```python
from build123d import *

# Parameters (mm, degrees)
P_IDAT_VYSUNUT_M1_DEPTH = 8
ZAOBLIT1_R              = 2


with BuildPart() as part:
    # Skica1 → Přidat vysunutím1 (new body)
    with BuildSketch(Plane.XY):
        with BuildLine():
            Line((1.2, 7.9), (1.2, 5.9))
            Line((1.2, 5.9), (3, 5.9))
            Line((3, 5.9), (3, 4.1))
            Line((3, 4.1), (1.2, 4.1))
            Line((1.2, 4.1), (1.2, -4.1))
            Line((1.2, -4.1), (3, -4.1))
            Line((3, -4.1), (3, -5.9))
            Line((3, -5.9), (1.2, -5.9))
            Line((1.2, -5.9), (1.2, -7.9))
            Line((1.2, -7.9), (-0.9, -7.9))
            Line((-0.9, -7.9), (-0.9, -9.7))
            Line((-0.9, -9.7), (-2.7, -9.7))
            Line((-2.7, -9.7), (-2.7, -7.9))
            Line((-2.7, -7.9), (-4.526252218, -7.9))
            ThreePointArc((-4.526252218, -7.9), (-4.233358999, -7.192893219), (-3.526252218, -6.9))
            ThreePointArc((-3.526252218, -6.9), (-2.970681985, -6.731469612), (-2.602372686, -6.282683432))
            Line((-2.602372686, -6.282683432), (0, 0))
            Line((0, 0), (-2.602372686, 6.282683432))
            ThreePointArc((-2.602372686, 6.282683432), (-2.970681985, 6.731469612), (-3.526252218, 6.9))
            ThreePointArc((-3.526252218, 6.9), (-4.233358999, 7.192893219), (-4.526252218, 7.9))
            Line((-4.526252218, 7.9), (-2.7, 7.9))
            Line((-2.7, 7.9), (-2.7, 9.7))
            Line((-2.7, 9.7), (-0.9, 9.7))
            Line((-0.9, 9.7), (-0.9, 7.9))
            Line((-0.9, 7.9), (1.2, 7.9))
        make_face()
    extrude(amount=P_IDAT_VYSUNUT_M1_DEPTH)

    # Zaoblit1
    zaoblit1_edges = [part.edges().sort_by_distance(p)[0] for p in [
        (0, 0, 4),
    ]]
    fillet(zaoblit1_edges, radius=ZAOBLIT1_R)


solid = part.part
```
For this review, take the finished solid that the model builds, in its own axes (mm). A direction names the side the tool comes from. Give positions to 0.01 mm unless a question says otherwise; leave off trailing zeros. Write each loop counter-clockwise with the first axis right and the second up, starting at its lowest first coordinate (ties: lowest second). Pieces come first, ordered by that corner, then holes.
Item 1: Take a section at A-A (x = 2.75). Give the boundary of the cut face in (y, z).
Item 2: Wall thickness on probe 1 along Y at (x, z) = (2.5, 1.5); probe 2 along Y at (x, z) = (0.25, 6.25); probe 3 along X at (y, z) = (-9, 1.5): over which ranges is each line inside the solid? List them lowest first.
Item 3: Take a section at B-B (z = 2.75). Give the boundary of the cut face in (x, y), and give its area (3 significant figures).
Item 4: Machinability: for faces 5 (the face through (1.2, 7, 4)), 6 (the face through (-2.7, -9, 4)), 7 (the face through (1.2, -7, 4)), 8 (the face through (-1.476, -3.563, 3.944)), which of the approach directions +Z, -Z, +X, -X, +Y, -Y give a long, thin tool a straight path to every point of the face, cutting with its end or side? Answer none if there is none.
Item 5: Insertion check: P1, Ø1.4, axis at x = 2, z = 5, coming from the +Y side; P2, Ø4, axis at x = 2, z = 2, coming from the -Y side; P3, Ø2, axis at y = 9, z = 5, coming from the -X side; P4, Ø4, axis at x = -3.5, z = 4.5, coming from the +Y side. Each pin has a flat end and moves straight along its axis. Give the tip position at first contact, or say it passes through.
Item 6: Take a section at D-D (y = -1). Give the boundary of the cut face in (x, z), and give its area (3 significant figures).
Item 7: Take a section at C-C (x = -3.25). Give the boundary of the cut face in (y, z).
Item 8: The part is to be moulded in two halves that separate along Y. For faces 1 (the face through (0, -7.9, 4)), 2 (the face through (1.2, 0, 4)), 3 (the face through (0, 0, 0)), 4 (the face through (-0.165, -0.011, 4.056)), say which applies: +Y half, -Y half, draft (parallel to the pull), parting line (faces both ways), or undercut.
Established:
1. outline: (-5.9, 0) - (-4.1, 0) - (-4.1, 8) - (-5.9, 8) - close; (4.1, 0) - (5.9, 0) - (5.9, 8) - (4.1, 8) - close
2. probe 1: y = -5.9 to -4.1, 4.1 to 5.9
2. probe 2: y = -7.9 to 7.9
2. probe 3: x = -2.7 to -0.9
3. outline: (-4.53, -7.9) - (-2.7, -7.9) - (-2.7, -9.7) - (-0.9, -9.7) - (-0.9, -7.9) - (1.2, -7.9) - (1.2, -5.9) - (3, -5.9) - (3, -4.1) - (1.2, -4.1) - (1.2, 4.1) - (3, 4.1) - (3, 5.9) - (1.2, 5.9) - (1.2, 7.9) - (-0.9, 7.9) - (-0.9, 9.7) - (-2.7, 9.7) - (-2.7, 7.9) - (-4.53, 7.9) arc R1 ccw to (-3.53, 6.9) arc R1 cw to (-2.6, 6.28) - (-0.32, 0.77) arc R2 cw to (-0.32, -0.77) - (-2.6, -6.28) arc R1 cw to (-3.53, -6.9) arc R1 ccw to start
3. area: 60.5 mm2
4. face 5: +Z, -Z, +X, +Y
4. face 6: +Z, -Z, -X, -Y
4. face 7: +Z, -Z, +X, -Y
4. face 8: +Z, -Z, -X
5. P1: stops at y = 5.9
5. P2: stops at y = -7.9
5. P3: stops at x = -2.7
5. P4: stops at y = 9.7
6. outline: (-0.41, 0) - (1.2, 0) - (1.2, 8) - (-0.41, 8) - close
6. area: 12.9 mm2
7. outline: (-7.9, 0) - (-6.86, 0) - (-6.86, 8) - (-7.9, 8) - close; (6.86, 0) - (7.9, 0) - (7.9, 8) - (6.86, 8) - close
8. face 1: -Y half
8. face 2: undercut
8. face 3: draft
8. face 4: undercut
